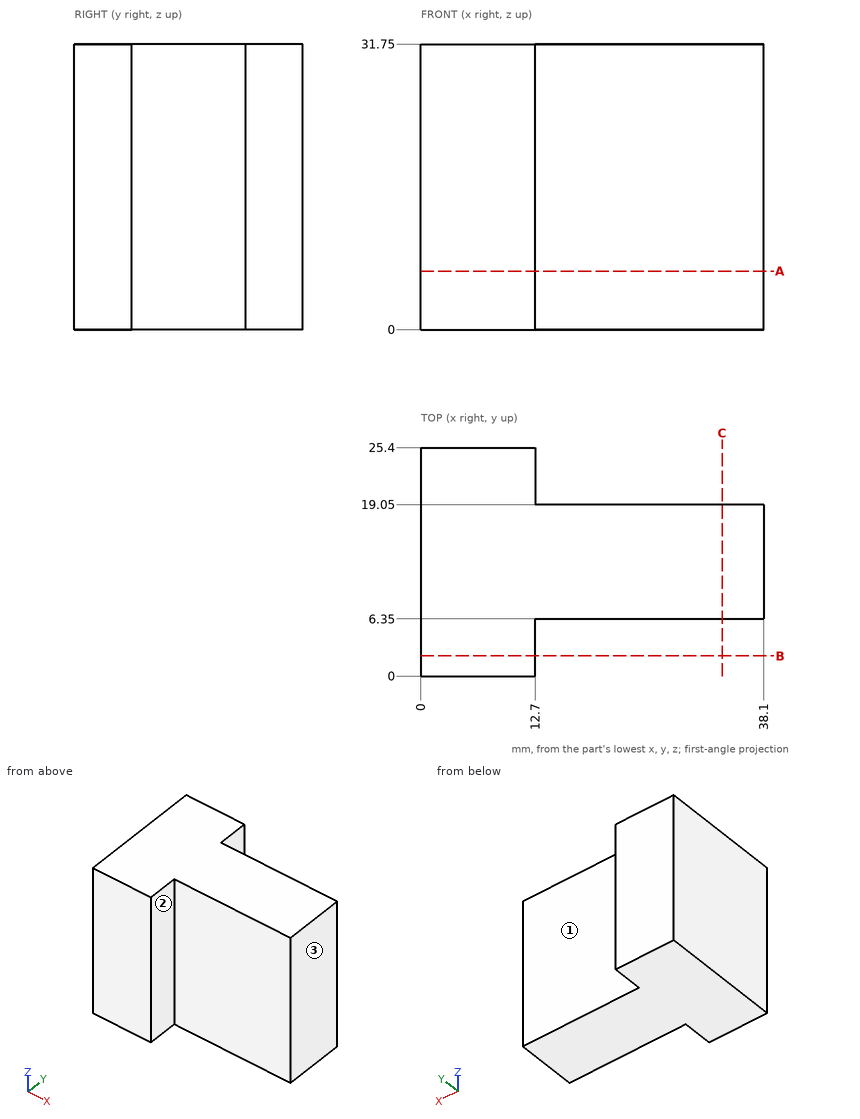
Study the drawing (mm; zero at the part's minimum x, y, z) and answer. A direction names the side the tool comes from. Coordinates: 2 decimals unless noted, no trailing zeros. Loops run counter-clockwise (first coordinate to the right, second up) from the corner with the lowest first, then second, coordinate; pieces in that order, holes last. Notation, with made-up numbers: M 75,-10.75 L 87,-10.75 A14 cw 87,11.25 Z; hole C 45.25,54.25 d8. An arc over 180 degrees is marked long. Answer as a JSON object with one key per item and string values. Group by question number.
Item 1: Section B-B (y = 2.25) is taken. Write down the section's boundary in (x, z), and give its area (3 significant figures).
Item 2: Each of these flat-tipped pins is pushed along its axis until it touches: P1, Ø1.9, axis at y = 2, z = 23, coming from the +X side; P2, Ø5, axis at x = 33, z = 4.5, coming from the -Y side; P3, Ø1, axis at x = 25.5, y = 5, coming from the -Z side. Where does it stop, or does it pass through?
Item 3: Section C-C (x = 33.5) is taken. Write down the section's boundary in (y, z), and give its area (3 significant figures).
Item 4: Consider L1, parallel to Y at x = 36.5, z = 18; L2, parallel to X at y = 22.5, z = 8. Determine where each line is inside the solid, lowest interval first.
Item 5: Which of the six approach directions +Z, -Z, +X, -X, +Y, -Y give full straight-line access (tool end or side, diameter ignored) to the marked faces 1, 2 and 3?
Item 6: Section A-A (z = 6.5) is taken. Write down the section's boundary in (x, y), and give its area (3 significant figures).
Solved:
{
 "1": {"outline": "M 0,0 L 12.7,0 L 12.7,31.75 L 0,31.75 Z", "area": "403 mm2"},
 "2": {"P1": "stops at x = 12.7", "P2": "stops at y = 6.35", "P3": "passes through"},
 "3": {"outline": "M 6.35,0 L 19.05,0 L 19.05,31.75 L 6.35,31.75 Z", "area": "403 mm2"},
 "4": {"L1": "y = 6.35 to 19.05", "L2": "x = 0 to 12.7"},
 "5": {"face 1": "+Z, -Z, +X, +Y", "face 2": "+Z, -Z, +X, -Y", "face 3": "+Z, -Z, +X, +Y, -Y"},
 "6": {"outline": "M 0,0 L 12.7,0 L 12.7,6.35 L 38.1,6.35 L 38.1,19.05 L 12.7,19.05 L 12.7,25.4 L 0,25.4 Z", "area": "645 mm2"}
}
